Part print with two shaded views. Sizes in mm from the minimum x, y, z corner. A direction names the side the tool comes from. Round coordinates to 2 decimals unless told otherwise and drop trailing zeros. Loops run counter-clockwise (first coordinate to the right, second up) from the corner with the lowest first, then second, coordinate; pieces in that order, holes last. Notation, with made-up numbers: (1, 88.5) -> (53, 88.5) arc R17 ccw to (53, 117.5) -> close; hole circle Ø11 at (-36.75, 79). An arc over 180 degrees is marked (long way). Use a Markdown table: item, result. Add a question column.
Item 1: Flat gauge pins, fed straight in: pin 1 (3 mm diameter, centred on y = 9.5, z = 76.5, fed in from +X); pin 2 (6 mm diameter, centred on y = 5.5, z = 85, fed in from +X); pin 3 (10 mm diameter, centred on x = 228.6, z = 127, fed in from -Y); pin 4 (1.9 mm diameter, centred on y = 2, z = 114, fed in from -X). Where does each tip first touch, or does it go through?
Item 2: Cut at A-A, the plane z = 25.4. List the corners of the cut face in (x, y), plus the area to 3 significant figures.
Item 3: Cut at B-B, the plane x = 127. List the corners of the cut face in (y, z), plus the area to 3 significant figures.
Item 4: Probe line 1 (Z direction, x = 228.6, y = 1.5); line 2 (Y direction, x = 162, z = 119); line 3 (Z direction, x = 92.5, y = 6.5). List the from-to ranges inside material, lowest first. Write a range as [from, to].
Item 5: Cut at C-C, the plane z = 124. List the corners of the cut face in (x, y).
Item 6: Which spindle directions (+Z, -Z, +X, -X, +Y, -Y) get a long thin tool onto all of the face, cutting with end or side? Do the marked faces 1 and 2. Say none if no direction does.
Item 7: Cut at D-D, the plane x = 50. List the corners of the cut face in (y, z), plus the area to 3 significant figures.
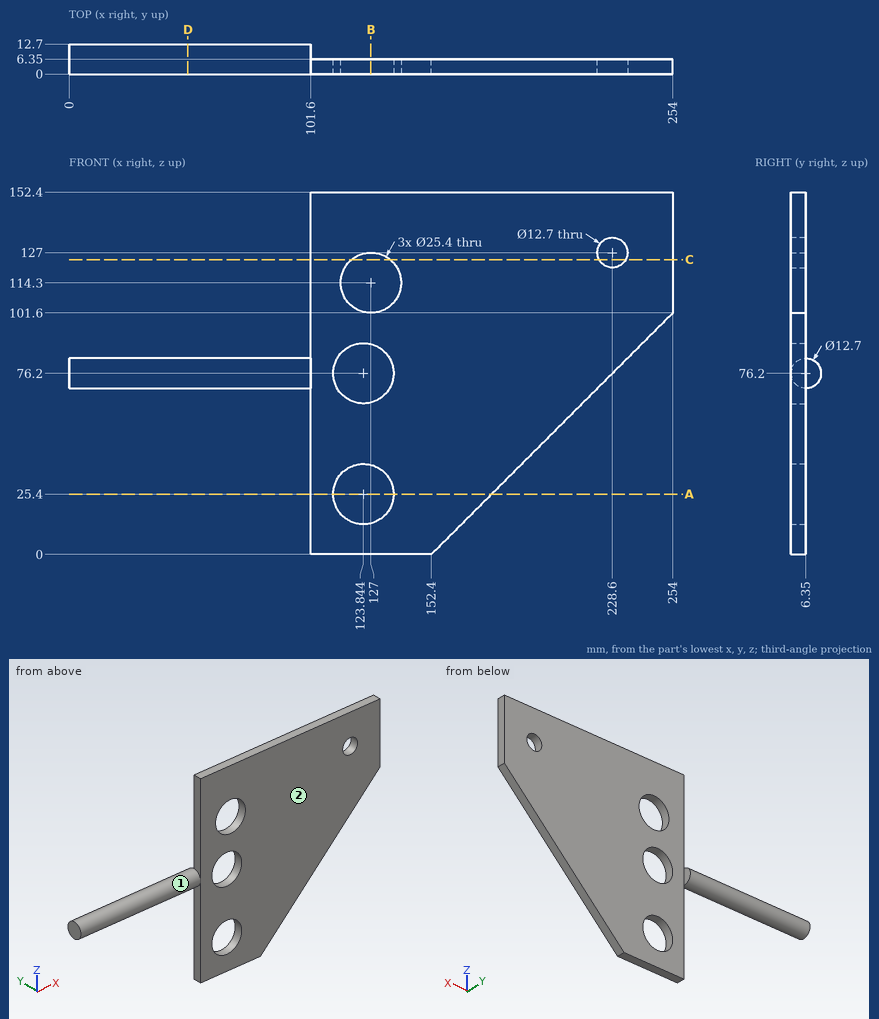
A:
| question | item | result |
|---|---|---|
| 1 | pin 1 | stops at x = 101.6 |
| 1 | pin 2 | stops at x = 240.4 |
| 1 | pin 3 | passes through |
| 1 | pin 4 | stops at x = 101.6 |
| 2 | outline | (101.6, 0) -> (111.14, 0) -> (111.14, 6.35) -> (101.6, 6.35) -> close; (136.54, 0) -> (177.8, 0) -> (177.8, 6.35) -> (136.54, 6.35) -> close |
| 2 | area | 323 mm^2 |
| 3 | outline | (0, 0) -> (6.35, 0) -> (6.35, 13.1) -> (0, 13.1) -> close; (0, 37.7) -> (6.35, 37.7) -> (6.35, 63.9) -> (0, 63.9) -> close; (0, 88.5) -> (6.35, 88.5) -> (6.35, 101.6) -> (0, 101.6) -> close; (0, 127) -> (6.35, 127) -> (6.35, 152.4) -> (0, 152.4) -> close |
| 3 | area | 494 mm^2 |
| 4 | line 1 | z = [76.2, 120.65], [133.35, 152.4] |
| 4 | line 2 | y = [0, 6.35] |
| 4 | line 3 | z = [69.85, 82.55] |
| 5 | outline | (101.6, 0) -> (118.8, 0) -> (118.8, 6.35) -> (101.6, 6.35) -> close; (135.2, 0) -> (223, 0) -> (223, 6.35) -> (135.2, 6.35) -> close; (234.2, 0) -> (254, 0) -> (254, 6.35) -> (234.2, 6.35) -> close |
| 6 | face 1 | -X |
| 6 | face 2 | +Z, -Z, +X, -X, -Y |
| 7 | outline | circle Ø12.7 at (6.35, 76.2) |
| 7 | area | 127 mm^2 |
